The model under review builds one solid part; all positions refer to its coordinate system, in mm. Face numbers are marked on the shaded views. A direction names the side the tool comes from. Coordinates: 2 decimals unless noted, no trailing zeros. Loops run counter-clockwise (first coordinate to the right, second up) from the corner with the lowest first, then second, coordinate; pieces in that order, holes last. Notation, with made-up numbers: M -36.5,72.25 L 10.5,72.25 A11 cw 10.5,87.25 Z; hole C -2,-5 d4. An arc over 180 degrees is marked long. Use CSV: the item, a comma, the result in double quotes. Start each with the question number.
1. Draft analysis for pull direction Y (two halves, no side actions). For the marked faces 4, 5 and 6, state which applies: +Y half, -Y half, draft (parallel to the pull), parting line (faces both ways), or undercut.
2. Add section C-C, the plane y = -4.25. Write out the cut boundary in (x, z), then the cut area to 3 significant figures.
3. Clearance check with flat-ended pins moving along their axes: P1, Ø3, axis at x = 0, z = 4.5, coming from the +Y side; P2, Ø0.7, axis at y = 6, z = -2.5, coming from the -X side; P3, Ø3.5, axis at y = 0.5, z = 1.5, coming from the +X side. State where each tip first meets the part, or that it passes through.
4. Add section A-A, the plane z = 0. Write out the cut boundary in (x, y).
5. Add section D-D, the plane z = 6.5. Write out the cut boundary in (x, y).
6. For L1, parallel to Z at x = 1.5, y = 4.5; L2, parallel to Y at x = 7.75, z = -6.5; L3, parallel to Z at x = 8, y = -7, list the stretches that pass through material, from the lowest coordinate up.
7. Tool access review of the marked faces 1, 2 and 3: name each direction out of +Z, -Z, +X, -X, +Y, -Y from which nothing blocks a thin tool from reaching the whole face with its end or side.
8. Add section B-B, the plane x = -0.5. Write out the cut boundary in (y, z).
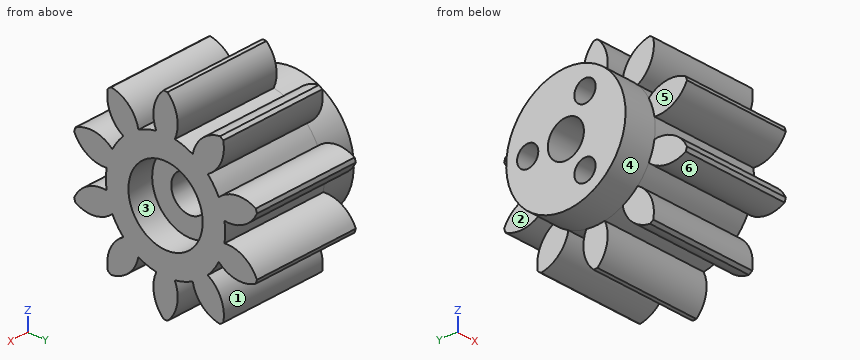
from build123d import *
from build123d.topology import SkipClean

# Parameters (mm, degrees)
BASPROSKE_W                                          = 10
BASPROSKE_H                                          = 9
TOOTHCUT_DEPTH                                       = 17.186414
TEETHCUTS_COUNT                                      = 10
SALIENTE_EXTRUIR2_START                              = 3
CROQUIS2_R                                           = 5.624
SALIENTE_EXTRUIR2_DEPTH                              = 3
REFRENTADO_PARA_TORNILLO_CON_CABEZA_TRON_D           = 3.4
REFRENTADO_PARA_TORNILLO_CON_CABEZA_TRON_CBORE_D     = 7
REFRENTADO_PARA_TORNILLO_CON_CABEZA_TRON_CBORE_DEPTH = 2.4
CROQUIS5_R                                           = 1
CORTAR_EXTRUIR1_DEPTH                                = 3


with BuildPart() as part:
    # BasProSke → Base-Revolve (revolve)
    with BuildSketch(Plane(origin=(0, 0, 0), x_dir=(1, 0, 0), z_dir=(0, 1, 0)), mode=Mode.PRIVATE) as base_revolve_sk:
        with Locations((5, 4.5)):
            Rectangle(BASPROSKE_W, BASPROSKE_H)
    revolve(base_revolve_sk.sketch.rotate(Axis((-10, 0, 0), (1, 0, 0)), 180), axis=Axis((-10, 0, 0), (1, 0, 0)))

    # TooCutSke → ToothCut (cut, through all)
    with BuildSketch(Plane(origin=(0, 0, 0), x_dir=(0, 0, -1), z_dir=(1, 0, 0))):
        with BuildLine():
            ThreePointArc((0.883878, 5.55411), (0, 5.624), (-0.883878, 5.55411))
            ThreePointArc((-0.883878, 5.55411), (-1.258246, 7.379188), (-2.637817, 8.631325))
            ThreePointArc((-2.637817, 8.631325), (0, 9.0254), (2.637817, 8.631325))
            ThreePointArc((2.637817, 8.631325), (1.258246, 7.379188), (0.883878, 5.55411))
        make_face()
    toothcut = extrude(amount=TOOTHCUT_DEPTH, mode=Mode.SUBTRACT)

    # TeethCuts: ToothCut ×10 about axis
    teethcuts_axis = Axis((0, 0, 0), (1, 0, 0))
    for i in range(1, TEETHCUTS_COUNT):
        add(toothcut.rotate(teethcuts_axis, i * 360 / TEETHCUTS_COUNT), mode=Mode.SUBTRACT)

    # Croquis2 → Saliente-Extruir2 (add)
    with SkipClean():  # the faces are left unmerged after this step: merging them gives an invalid solid
        with BuildSketch(Plane.ZY.offset(SALIENTE_EXTRUIR2_START)):
            Circle(CROQUIS2_R)
        extrude(amount=-SALIENTE_EXTRUIR2_DEPTH)

    # Refrentado para tornillo con cabeza troncocónica de M31 (through all)
    with Locations(Plane(origin=(10, 0, 0), x_dir=(0, 0, -1), z_dir=(1, 0, 0))):
        with Locations((0, 0)):
            CounterBoreHole(REFRENTADO_PARA_TORNILLO_CON_CABEZA_TRON_D / 2, REFRENTADO_PARA_TORNILLO_CON_CABEZA_TRON_CBORE_D / 2, REFRENTADO_PARA_TORNILLO_CON_CABEZA_TRON_CBORE_DEPTH)

    # Croquis5 → Cortar-Extruir1 (cut)
    with SkipClean():  # the faces are left unmerged after this step: merging them gives an invalid solid
        with BuildSketch(Plane.ZY.offset(3)):
            with Locations((0, 3.6)):
                Circle(CROQUIS5_R)
            with Locations((3.117691, -1.8)):
                Circle(CROQUIS5_R)
            with Locations((-3.117691, -1.8)):
                Circle(CROQUIS5_R)
        extrude(amount=-CORTAR_EXTRUIR1_DEPTH, mode=Mode.SUBTRACT)


solid = part.part
Computed:
1,face 4,"parting line"
1,face 5,"draft"
1,face 6,"undercut"
2,outline,"M -3,-3.68 L 10,-3.68 L 10,3.68 L -3,3.68 Z; M 0,-7.14 L 10,-7.14 L 10,-4.16 L 0,-4.16 Z; M 0,4.16 L 10,4.16 L 10,7.14 L 0,7.14 Z"
2,area,"155 mm^2"
3,P1,"stops at y = 8.42"
3,P2,"stops at x = 0"
3,P3,"stops at x = 7.6"
4,outline,"M -3,-5.62 L 10,-5.62 L 10,-3.5 L 7.6,-3.5 L 7.6,-1.7 L -3,-1.7 Z; M -3,1.7 L 7.6,1.7 L 7.6,3.5 L 10,3.5 L 10,5.62 L -3,5.62 L -3,4.6 L 0,4.6 L 0,2.6 L -3,2.6 Z"
5,outline,"M 0,-5.5 L 10,-5.5 L 10,-3.34 L 0,-3.34 Z; M 0,-1.13 L 10,-1.13 L 10,1.13 L 0,1.13 Z; M 0,3.34 L 10,3.34 L 10,5.5 L 0,5.5 Z"
6,L1,"z = -7.24 to -4.36, -3.37 to 3.37, 4.36 to 7.24"
6,L2,"y = -5.5 to -3.34, -1.13 to 1.13, 3.34 to 5.5"
6,L3,"z = -3.34 to -1.08, 1.08 to 3.34"
7,face 1,"+X, -X, +Y"
7,face 2,"-Z, -X, +Y"
7,face 3,"+X"
8,outline,"C 0,0 d11.25; hole C -1.8,-3.12 d2; hole C -1.8,3.12 d2; hole C 0,0 d3.4; hole C 3.6,0 d2"
